Check sheet for the drawn part. Datum: minimum x, y, z corner. Units: mm. Give positions to 0.01 mm unless a question says otherwise; leave off trailing zeros. Write each loop counter-clockwise with the first axis right and the second up, starting at its lowest first coordinate (ties: lowest second). Pieces come first, ordered by that corner, then holes. Notation, with made-up numbers: M 41,-24 L 68,-24 A13 ccw 68,0 Z; hole C 56,65.5 d6. An arc over 180 degrees is marked long. Use CSV: the item, a comma, the result in double quotes. Start each with the question number.
1. Scan lines: line 1 (Y direction, x = 12.7, z = 26.5) (3 decimals); line 2 (X direction, y = 50.8, z = 16.5) (3 decimals); line 3 (Y direction, x = 14.25, z = 35.5). Record each from-to range of solid material in increasing order.
2. Cross-section at B-B, the plane z = 39. Enter the section's corners in (x, y) (3 decimals).
3. Cross-section at C-C, the plane x = 6. Enter the section's corners in (y, z), and give its area (3 significant figures).
4. Cross-section at A-A, the plane x = 12.7. Enter the section's corners in (y, z) (3 decimals), and give its area (3 significant figures).
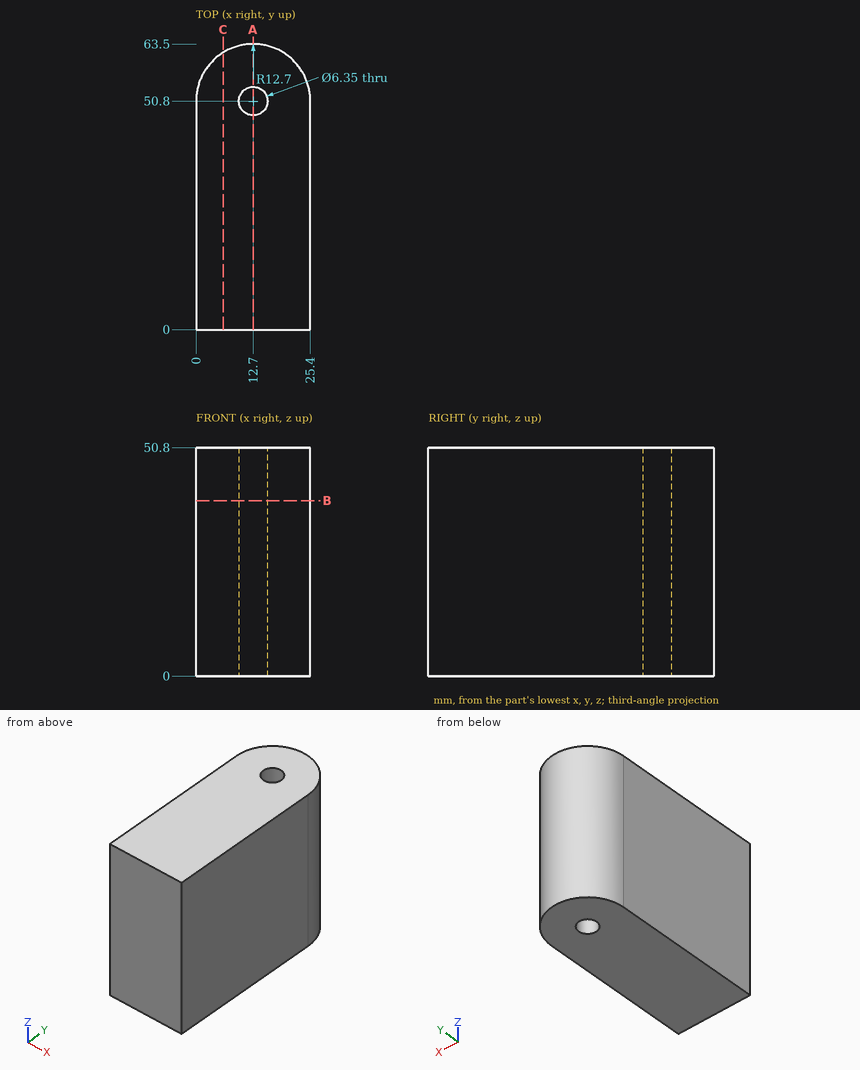
Worked answers:
1,line 1,"y = 0 to 47.625, 53.975 to 63.5"
1,line 2,"x = 0 to 9.525, 15.875 to 25.4"
1,line 3,"y = 0 to 48.03, 53.57 to 63.41"
2,outline,"M 0,0 L 25.4,0 L 25.4,50.8 A12.7 ccw 0,50.8 Z; hole C 12.7,50.8 d6.35"
3,outline,"M 0,0 L 61.59,0 L 61.59,50.8 L 0,50.8 Z"
3,area,"3,130 mm^2"
4,outline,"M 0,0 L 47.625,0 L 47.625,50.8 L 0,50.8 Z; M 53.975,0 L 63.5,0 L 63.5,50.8 L 53.975,50.8 Z"
4,area,"2,900 mm^2"
